from build123d import *

# Parameters (mm, degrees)
BOSS_EXTRUDE1_DEPTH     = 17.5
CUT_EXTRUDE1_DEPTH      = 85.085150294
CUT_EXTRUDE1_DEPTH_BACK = 85.085150294
SKETCH2_R               = 1.98501
FILLET1_R               = 2


with BuildPart() as part:
    # Sketch1 → Boss-Extrude1 (new, symmetric)
    with BuildSketch(Plane.XY):
        Polygon((-39.75, -65), (-39.75, 72), (39.75, 72), (39.75, -65), (32.75, -65), (32.75, 65), (-32.75, 65), (-32.75, -65), align=None)
    extrude(amount=BOSS_EXTRUDE1_DEPTH, both=True)

    # Sketch2 → Cut-Extrude1 (cut, two sides: drawn at the far end of the back side and taken through both)
    with BuildSketch(Plane(origin=(0, 0, 0), x_dir=(0, 0, -1), z_dir=(1, 0, 0)).offset(-CUT_EXTRUDE1_DEPTH_BACK)):
        with Locations((-7.5, -55)):
            Circle(SKETCH2_R)
        with Locations((7.5, -55)):
            Circle(SKETCH2_R)
    extrude(amount=CUT_EXTRUDE1_DEPTH + CUT_EXTRUDE1_DEPTH_BACK, mode=Mode.SUBTRACT)

    # Fillet1
    fillet1_edges = [part.edges().sort_by_distance(p)[0] for p in [
        (-39.75, 72, 0),
        (39.75, 72, 0),
    ]]
    fillet(fillet1_edges, radius=FILLET1_R)


solid = part.part
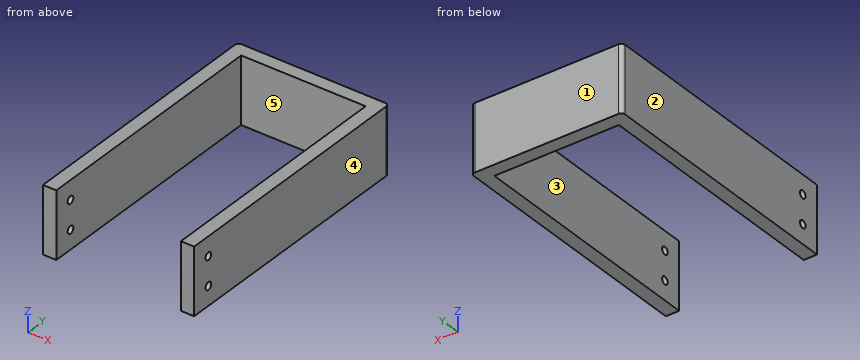
Design review of the part built by this model. Coordinates are the model's own, in mm. Face numbers are marked on the shaded views. A direction names the side the tool comes from. Coordinates: 2 decimals unless noted, no trailing zeros. Order: outer loops, then holes, each group sorted by start corner. A loop starts at its lowest first (then second) coordinate and runs counter-clockwise, first axis right, second up. Notation, with made-up numbers: (20, 3) -> (64, 3) arc R14 cw to (64, 17) -> close; hole circle Ø9 at (5.25, 37). An arc over 180 degrees is marked (long way). Use one line per item in the form item = value. Start each with the question number.
(1) For probe 1 along Z at (x, y) = (-37, -55); probe 2 along Y at (x, z) = (34.5, 7.5); probe 3 along X at (y, z) = (32, 4), list the stretches that pass through material, from the lowest coordinate up.
(2) The part is to be moulded in two halves that separate along X. For the marked faces 1, 2 and 3, say which applies: +X half, -X half, draft (parallel to the pull), parting line (faces both ways), or undercut.
(3) Add section A-A on y = 58.5. State the section outline as (x, z) points.
(4) Add section D-D on z = 1. State the section outline as (x, y) points.
(5) Add section B-B on z = 7.5. State the section outline as (x, y) points, plus the area to 3 significant figures.
(6) For the marked faces 4 and 5, list the 3-axis set-ups (+Z, -Z, +X, -X, +Y, -Y) from which the entire face can be reached by the end or side of a thin tool; tool diameter is ignored.
(7) Add section C-C on y = -55. State the section outline as (x, z) points (3 decimals), plus the area to 3 significant figures.
Answer block:
q1.probe_1 = -17.5 to -9.49, -5.51 to 5.51, 9.49 to 17.5
q1.probe_2 = -65 to -56.99, -53.01 to 72
q1.probe_3 = -39.75 to -32.75, 32.75 to 39.75
q2.face_1 = draft
q2.face_2 = -X half
q2.face_3 = undercut
q3.outline = (-39.75, -17.5) -> (-32.75, -17.5) -> (-32.75, 17.5) -> (-39.75, 17.5) -> close; (32.75, -17.5) -> (39.75, -17.5) -> (39.75, 17.5) -> (32.75, 17.5) -> close
q4.outline = (-39.75, -65) -> (-32.75, -65) -> (-32.75, 65) -> (32.75, 65) -> (32.75, -65) -> (39.75, -65) -> (39.75, 70) arc R2 ccw to (37.75, 72) -> (-37.75, 72) arc R2 ccw to (-39.75, 70) -> close
q5.outline = (-39.75, -65) -> (-32.75, -65) -> (-32.75, -56.99) -> (-39.75, -56.99) -> close; (-39.75, -53.01) -> (-32.75, -53.01) -> (-32.75, 65) -> (32.75, 65) -> (32.75, -53.01) -> (39.75, -53.01) -> (39.75, 70) arc R2 ccw to (37.75, 72) -> (-37.75, 72) arc R2 ccw to (-39.75, 70) -> close; (32.75, -65) -> (39.75, -65) -> (39.75, -56.99) -> (32.75, -56.99) -> close
q5.area = 2,320 mm²
q6.face_4 = +Z, -Z, +X, +Y, -Y
q6.face_5 = +Z, -Z, -Y
q7.outline = (-39.75, -17.5) -> (-32.75, -17.5) -> (-32.75, -9.485) -> (-39.75, -9.485) -> close; (-39.75, -5.515) -> (-32.75, -5.515) -> (-32.75, 5.515) -> (-39.75, 5.515) -> close; (-39.75, 9.485) -> (-32.75, 9.485) -> (-32.75, 17.5) -> (-39.75, 17.5) -> close; (32.75, -17.5) -> (39.75, -17.5) -> (39.75, -9.485) -> (32.75, -9.485) -> close; (32.75, -5.515) -> (39.75, -5.515) -> (39.75, 5.515) -> (32.75, 5.515) -> close; (32.75, 9.485) -> (39.75, 9.485) -> (39.75, 17.5) -> (32.75, 17.5) -> close
q7.area = 379 mm²
